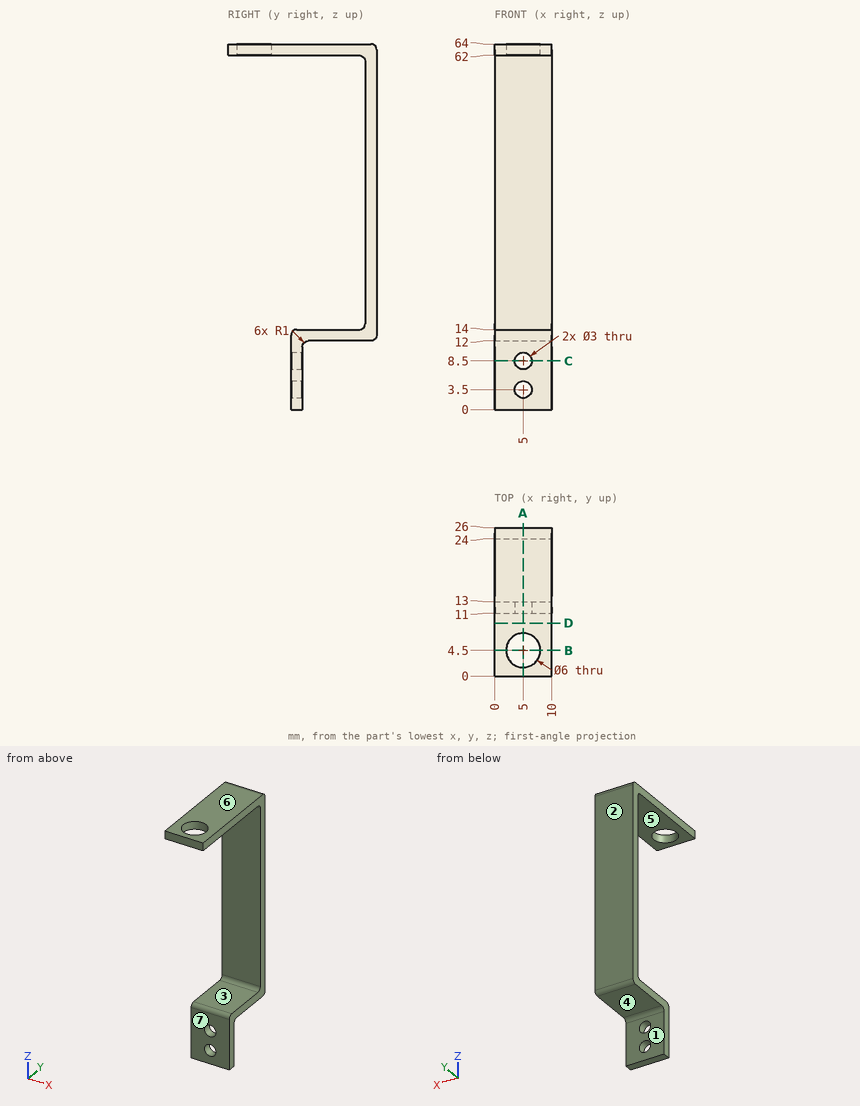
Print and shaded views of the part. All mm, measured from the part's lowest x, y and z. A direction names the side the tool comes from. Coordinates: 2 decimals unless noted, no trailing zeros. Loops run counter-clockwise (first coordinate to the right, second up) from the corner with the lowest first, then second, coordinate; pieces in that order, holes last. Notation, with made-up numbers: (-8, -18.75) - (-2, -18.75) arc R23 ccw to (-2, 18.25) - close; hole circle Ø2 at (-2, 73.25). An arc over 180 degrees is marked (long way). Write item = value, one per line. Start each with the question number.
Item 1: Cut at D-D, the plane y = 9.25. Give the cut face in (x, z).
Item 2: Cut at A-A, the plane x = 5. Give the cut face in (y, z), and give its area (3 significant figures).
Item 3: Flat gauge pins, fed straight in: pin 1 Ø5 at (x, y) = (7.5, 22) entering from -Z; pin 2 Ø4 at (x, y) = (8.5, 4.5) entering from -Z; pin 3 Ø4 at (x, z) = (5, 56.5) entering from -Y. Where does each tip first touch, or does it go through?
Item 4: Cut at C-C, the plane z = 8.5. Give the cut face in (x, y), and give its area (3 significant figures).
Item 5: 3-axis set-ups, long thin cutter, end or side, ignore diameter. For the marked faces 1, 2 and 3: which of +Z, -Z, +X, -X, +Y, -Y reach the whole face in a straight line?
Item 6: Cut at B-B, the plane y = 4.5. Give the cut face in (x, z).
Item 7: Wall check: L1, parallel to X at y = 12.2, z = 8.5; L2, parallel to Z at x = 1, y = 19.75; L3, parallel to Y at x = 1, z = 3.5. Give the ranges that are in metal, low to high. Write a range as from..to.
Item 8: Mould opens along Z. For the marked faces 4, 5, 6 and 7 say: released by +Z, released by -Z, zero draft, split by the parting line, or undercut.
The answers:
q1.outline = (0, 62) - (10, 62) - (10, 64) - (0, 64) - close
q2.outline = (0, 62) - (1.5, 62) - (1.5, 64) - (0, 64) - close; (7.5, 62) - (23, 62) arc R1 cw to (24, 61) - (24, 15) arc R1 cw to (23, 14) - (12, 14) arc R1 ccw to (11, 13) - (11, 10) - (13, 10) - (13, 11) arc R1 cw to (14, 12) - (25, 12) arc R1 ccw to (26, 13) - (26, 63) arc R1 ccw to (25, 64) - (7.5, 64) - close; (11, 0) - (13, 0) - (13, 2) - (11, 2) - close; (11, 5) - (13, 5) - (13, 7) - (11, 7) - close
q2.area = 178 mm2
q3.pin_1 = 12
q3.pin_2 = 62
q3.pin_3 = 24
q4.outline = (0, 11) - (3.5, 11) - (3.5, 13) - (0, 13) - close; (6.5, 11) - (10, 11) - (10, 13) - (6.5, 13) - close
q4.area = 14.0 mm2
q5.face_1 = -Z, +X, -X, +Y
q5.face_2 = +Z, -Z, +X, -X, +Y
q5.face_3 = +X, -X, -Y
q6.outline = (0, 62) - (2, 62) - (2, 64) - (0, 64) - close; (8, 62) - (10, 62) - (10, 64) - (8, 64) - close
q7.L1 = 0..3.5, 6.5..10
q7.L2 = 12..14, 62..64
q7.L3 = 11..13
q8.face_4 = released by -Z
q8.face_5 = undercut
q8.face_6 = released by +Z
q8.face_7 = zero draft
